CAD build for the part. Positions are in the model's coordinates, mm. Face numbers are marked on the shaded views. A direction names the side the tool comes from. Round coordinates to 2 decimals unless told otherwise and drop trailing zeros. Loops run counter-clockwise (first coordinate to the right, second up) from the corner with the lowest first, then second, coordinate; pieces in that order, holes last.
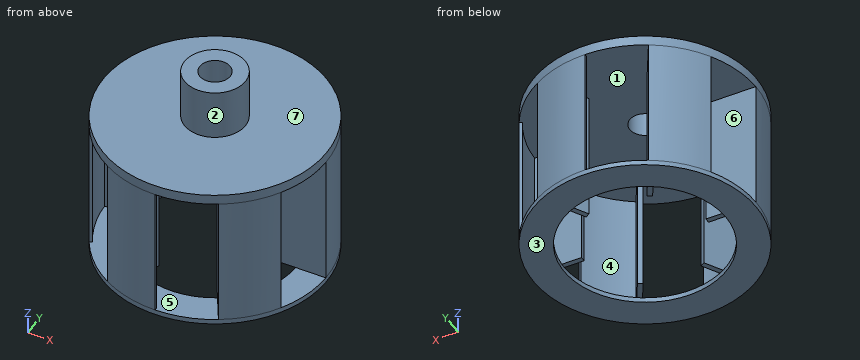
from build123d import *
from build123d.topology import SkipClean

# Parameters (mm, degrees)
BOSS_EXTRUDE1_START = 6.5
BOSS_EXTRUDE1_DEPTH = 6.5
BOSS_EXTRUDE2_START = 0.25
SKETCH3_R           = 5.5
SKETCH3_R_2         = 4
BOSS_EXTRUDE2_DEPTH = 0.25


with BuildPart() as part:
    # Sketch1 → Revolve1 (revolve)
    with BuildSketch(Plane(origin=(0, 0, 0), x_dir=(1, 0, 0), z_dir=(0, 1, 0)), mode=Mode.PRIVATE) as revolve1_sk:
        Polygon((5.5, 0.5), (0.75, 0.5), (0.75, -2.5), (1.5, -2.5), (1.5, 0), (5.5, 0), align=None)
    revolve(revolve1_sk.sketch.rotate(Axis((0, 0, -4.303790718), (0, 0, 1)), 180), axis=Axis((0, 0, -4.303790718), (0, 0, 1)))

    # Sketch2 → Boss-Extrude1 (add)
    with SkipClean():  # the faces are left unmerged after this step: merging them gives an invalid solid
        with BuildSketch(Plane(origin=(0, 0, -0.5), x_dir=(-1, 0, 0), z_dir=(0, 0, -1)).offset(BOSS_EXTRUDE1_START)):
            with BuildLine():
                Line((5.5, 0), (3.02, 0))
                Line((3.02, 0), (3.02, -0.25))
                Line((3.02, -0.25), (5.344155686, -0.25))
                ThreePointArc((5.344155686, -0.25), (5.133930465, -1.505077401), (4.63323591, -2.675))
                Line((4.63323591, -2.675), (4.763139721, -2.75))
                ThreePointArc((4.763139721, -2.75), (5.312592045, -1.423504748), (5.5, 0))
            make_face()
            with BuildLine():
                Line((2.75, -4.763139721), (1.51, -2.615396719))
                Line((1.51, -2.615396719), (1.293493649, -2.740396719))
                Line((1.293493649, -2.740396719), (2.455571492, -4.753174586))
                ThreePointArc((2.455571492, -4.753174586), (1.263529969, -5.198652904), (0, -5.35))
                Line((0, -5.35), (0, -5.5))
                ThreePointArc((0, -5.5), (1.423504748, -5.312592045), (2.75, -4.763139721))
            make_face()
            with BuildLine():
                Line((-2.75, -4.763139721), (-1.51, -2.615396719))
                Line((-1.51, -2.615396719), (-1.726506351, -2.490396719))
                Line((-1.726506351, -2.490396719), (-2.888584194, -4.503174586))
                ThreePointArc((-2.888584194, -4.503174586), (-3.870400496, -3.693575503), (-4.63323591, -2.675))
                Line((-4.63323591, -2.675), (-4.763139721, -2.75))
                ThreePointArc((-4.763139721, -2.75), (-3.889087297, -3.889087297), (-2.75, -4.763139721))
            make_face()
            with BuildLine():
                Line((-5.5, 0), (-3.02, 0))
                Line((-3.02, 0), (-3.02, 0.25))
                Line((-3.02, 0.25), (-5.344155686, 0.25))
                ThreePointArc((-5.344155686, 0.25), (-5.133930465, 1.505077401), (-4.63323591, 2.675))
                Line((-4.63323591, 2.675), (-4.763139721, 2.75))
                ThreePointArc((-4.763139721, 2.75), (-5.312592045, 1.423504748), (-5.5, 0))
            make_face()
            with BuildLine():
                Line((-2.75, 4.763139721), (-1.51, 2.615396719))
                Line((-1.51, 2.615396719), (-1.293493649, 2.740396719))
                Line((-1.293493649, 2.740396719), (-2.455571492, 4.753174586))
                ThreePointArc((-2.455571492, 4.753174586), (-1.263529969, 5.198652904), (0, 5.35))
                Line((0, 5.35), (0, 5.5))
                ThreePointArc((0, 5.5), (-1.423504748, 5.312592045), (-2.75, 4.763139721))
            make_face()
            with BuildLine():
                Line((2.75, 4.763139721), (1.51, 2.615396719))
                Line((1.51, 2.615396719), (1.726506351, 2.490396719))
                Line((1.726506351, 2.490396719), (2.888584194, 4.503174586))
                ThreePointArc((2.888584194, 4.503174586), (3.870400496, 3.693575503), (4.63323591, 2.675))
                Line((4.63323591, 2.675), (4.763139721, 2.75))
                ThreePointArc((4.763139721, 2.75), (3.889087297, 3.889087297), (2.75, 4.763139721))
            make_face()
        extrude(amount=-BOSS_EXTRUDE1_DEPTH)

    # Sketch3 → Boss-Extrude2 (add)
    with SkipClean():  # the faces are left unmerged after this step: merging them gives an invalid solid
        with BuildSketch(Plane(origin=(0, 0, -7), x_dir=(-1, 0, 0), z_dir=(0, 0, -1)).offset(BOSS_EXTRUDE2_START)):
            Circle(SKETCH3_R)
            Circle(SKETCH3_R_2, mode=Mode.SUBTRACT)
        extrude(amount=-BOSS_EXTRUDE2_DEPTH)


solid = part.part
Item 1: Cut at B-B (z = -4.5). State how many separate pieces and enclosed holes the cut face has, plus the area to 3 significant figures.
Verdict:
separate pieces: 6
enclosed holes: 0
area: 6.05 mm2
Item 2: Mould opens along Y. For the marked faces 1, 2, 3 and 4 say: released by +Y, released by -Y, zero draft, split by the parting line, or undercut.
Verdict:
face 1: undercut
face 2: split by the parting line
face 3: zero draft
face 4: undercut
Item 3: Cut at A-A (y = 1.25). List the corners of the cut face in (x, z).
Verdict:
outline: (-5.36, -7.25) - (-3.8, -7.25) - (-3.8, -7) - (-5.36, -7) - close; (-5.36, -0.5) - (5.2, -0.5) - (5.2, -7) - (3.8, -7) - (3.8, -7.25) - (5.36, -7.25) - (5.36, 0) - (0.83, 0) - (0.83, 2.5) - (-0.83, 2.5) - (-0.83, 0) - (-5.36, 0) - close
Item 4: 3-axis set-ups, long thin cutter, end or side, ignore diameter. For the marked faces 5, 6 and 7: which of +Z, -Z, +X, -X, +Y, -Y reach the whole face in a straight line?
Verdict:
face 5: none
face 6: -X
face 7: +Z
Item 5: Flat gauge pins, fed straight in: P1, Ø2, axis at x = -1, y = 4.5, coming from the +Z side; P2, Ø0.6, axis at x = 2, y = -3, coming from the -Z side; P3, Ø2, axis at x = 3.5, z = -5.5, coming from the -Y side; P4, Ø2, axis at x = 1.5, y = 1.5, coming from the +Z side. Where does each tip first touch, or does it go through?
Verdict:
P1: stops at z = 0
P2: stops at z = -7
P3: stops at y = -4.76
P4: stops at z = 2.5
Item 6: Wall check: L1, parallel to Y at x = 0, z = 0.2; L2, parallel to Z at x = -4.25, y = -2.25; L3, parallel to Y at x = 0, z = -7.2. Give the ranges that are in metal, low to high.
Verdict:
L1: y = -1.5 to -0.75, 0.75 to 1.5
L2: z = -7.25 to -7, -0.5 to 0
L3: y = -5.5 to -4, 4 to 5.5
